```python
from build123d import *

# Parameters (mm, degrees)
F0_R     = 0.5
F0_R_2   = 1.5
F0_R_3   = 2.5
F0_W     = 25
F0_H     = 14
F1_DEPTH = 4.4
F2_W     = 3.5
F2_H     = 9.5
F3_DEPTH = 8.6
F5_DEPTH = 3.5
F7_DEPTH = 7.6


with BuildPart() as f1:
    # F0 (on Top) → F1 (new body)
    with BuildSketch(Plane.XY):
        with BuildLine():
            Line((42.5, 44), (11.5, 44))
            ThreePointArc((11.5, 44), (3.368272, 40.631728), (0, 32.5))
            Line((0, 32.5), (0, 13.464194))
            ThreePointArc((0, 13.464194), (0.042012, 13.007801), (0.166636, 12.566746))
            Line((0.166636, 12.566746), (4.013814, 2.564084))
            ThreePointArc((4.013814, 2.564084), (5.482651, 0.702754), (7.747196, 0))
            Line((7.747196, 0), (40.5, 0))
            ThreePointArc((40.5, 0), (47.571068, 2.928932), (50.5, 10))
            Line((50.5, 10), (50.5, 36))
            ThreePointArc((50.5, 36), (48.156854, 41.656854), (42.5, 44))
        make_face()
        with Locations((10.5, 10.5)):
            Circle(F0_R, mode=Mode.SUBTRACT)
        with Locations((2.671147, 14.3)):
            Circle(F0_R_2, mode=Mode.SUBTRACT)
        with Locations((47.660035, 15.3)):
            Circle(F0_R_2, mode=Mode.SUBTRACT)
        with Locations((11.5, 32.5)):
            Circle(F0_R_3, mode=Mode.SUBTRACT)
        with Locations((34.5, 31.25)):
            Rectangle(F0_W, F0_H, mode=Mode.SUBTRACT)
        with Locations((30.8, 41.314212)):
            Circle(F0_R_2, mode=Mode.SUBTRACT)
    extrude(amount=F1_DEPTH)

    # F2 (on face) → F3 (join)
    with BuildSketch(Plane.XY.offset(4.4)):
        with Locations((48.75, 31.25)):
            Rectangle(F2_W, F2_H)
    extrude(amount=F3_DEPTH)

    # F4 (on face) → F5 (cut, through all)
    with BuildSketch(Plane.YZ.offset(50.5)):
        with BuildLine():
            Line((33.64583, 13), (28.85417, 13))
            ThreePointArc((28.85417, 13), (31.25, 8.9), (33.64583, 13))
        make_face()
        with BuildLine():
            Line((26.5, 13), (26.5, 4.4))
            Line((26.5, 4.4), (27, 10.7))
            Line((27, 10.7), (27.6, 10.7))
            ThreePointArc((27.6, 10.7), (27.809999, 11.920203), (28.415833, 13))
            Line((28.415833, 13), (26.5, 13))
        make_face()
        with BuildLine():
            ThreePointArc((34.084167, 13), (34.690001, 11.920203), (34.9, 10.7))
            Line((34.9, 10.7), (35.5, 10.7))
            Line((35.5, 10.7), (36, 4.4))
            Line((36, 4.4), (36, 13))
            Line((36, 13), (34.084167, 13))
        make_face()
    extrude(amount=-F5_DEPTH, mode=Mode.SUBTRACT)

    # F6 (on face) → F7 (join)
    with BuildSketch(Plane.XY.offset(4.4)):
        with BuildLine():
            Line((27.5, 7.5), (27.5, 0))
            Line((27.5, 0), (40.5, 0))
            ThreePointArc((40.5, 0), (42.017577, 0.115823), (43.5, 0.460608))
            Line((43.5, 0.460608), (43.5, 7.5))
            Line((43.5, 7.5), (27.5, 7.5))
        make_face()
    extrude(amount=F7_DEPTH)


solid = f1.part
```
Verification items for the finished model (mm, model axes). A direction names the side the tool comes from. Coordinates: 2 decimals unless noted, no trailing zeros. Write each loop counter-clockwise with the first axis right and the second up, starting at its lowest first coordinate (ties: lowest second). Pieces come first, ordered by that corner, then holes. Notation, with made-up numbers: M 27.5,76 L 53.5,76 A19 ccw 53.5,94 Z; hole C -3.5,20 d3. An arc over 180 degrees is marked long. One line per item, written item: value.
Item 1: Section check C-C, the plane z = 9.5. Record the boundary of the cut face in (x, y), plus the area to 3 significant figures.
Check sheet entries:
outline: M 27.5,0 L 40.5,0 A10 ccw 43.5,0.46 L 43.5,7.5 L 27.5,7.5 Z; M 47,26.9 L 50.5,26.9 L 50.5,29.54 L 47,29.54 Z; M 47,32.96 L 50.5,32.96 L 50.5,35.6 L 47,35.6 Z
area: 138 mm^2
Item 2: Section check B-B, the plane z = 5. Record the boundary of the cut face in (x, y).
Check sheet entries:
outline: M 27.5,0 L 40.5,0 A10 ccw 43.5,0.46 L 43.5,7.5 L 27.5,7.5 Z; M 47,26.55 L 50.5,26.55 L 50.5,35.95 L 47,35.95 Z
Item 3: Section check D-D, the plane x = 38. Record the boundary of the cut face in (y, z).
Check sheet entries:
outline: M 0,0 L 24.25,0 L 24.25,4.4 L 7.5,4.4 L 7.5,12 L 0,12 Z; M 38.25,0 L 44,0 L 44,4.4 L 38.25,4.4 Z
Item 4: Access from +Z, -Z, +X, -X, +Y, -Y to the whole of each face (thin tool, end or side, straight path). Record for faces 1 (the flat face through (27, 44, 2)), 2 (the flat face through (43.5, 4, 8)), 3 (the flat face through (36, 7.5, 8)), 4 (the flat face through (34, 38.25, 2)).
Check sheet entries:
face 1: +Z, -Z, +X, -X, +Y
face 2: +Z, +X, +Y, -Y
face 3: +Z, +X, -X, +Y
face 4: +Z, -Z
Item 5: Scan lines: line 1 along X through (y, z) = (28, 4.25); line 2 along Y through (x, z) = (34.5, 3); line 3 along X through (y, z) = (32, 1.5). Record each from-to range of solid material in increasing order.
Check sheet entries:
line 1: x = 0 to 22, 47 to 50.5
line 2: y = 0 to 24.25, 38.25 to 44
line 3: x = 0 to 9.05, 13.95 to 22, 47 to 50.5
Item 6: Mould release check, pull along X, two halves, no side actions. Record for faces 5 (the flat face through (28, 0, 5)), 6 (the flat face through (27.5, 4, 8)), 7 (the cylindrical face through (48.219, 41.594, 2.169)), 8 (the flat face through (47, 31, 5)): pulls with the +X half, pulls with the -X half, needs draft (parallel to the pull), parting line crosses it, or undercut.
Check sheet entries:
face 5: needs draft
face 6: pulls with the -X half
face 7: pulls with the +X half
face 8: undercut
Item 7: Gauge pin test, flat ends, axial feed: pin 1 Ø5 at (x, z) = (44, 11) entering from +Y; pin 2 Ø2 at (y, z) = (4.5, 9) entering from +X; pin 3 Ø10 at (x, y) = (40, 38.5) entering from +Z. Record the tip position at first contact, or that the pin passes through.
Check sheet entries:
pin 1: stops at y = 7.5
pin 2: stops at x = 43.5
pin 3: stops at z = 4.4
Item 8: Section check A-A, the plane x = 13. Record the boundary of the cut face in (y, z).
Check sheet entries:
outline: M 0,0 L 30.5,0 L 30.5,4.4 L 0,4.4 Z; M 34.5,0 L 44,0 L 44,4.4 L 34.5,4.4 Z
